Can you work these out from the model? Positions are in its coordinate system, mm. A direction names the side the tool comes from. Round coordinates to 2 decimals unless told otherwise and drop trailing zeros. Write each loop counter-clockwise with the first axis right and the second up, starting at its lowest first coordinate (ties: lowest second). Pieces come first, ordered by that corner, then holes.
Q1. Please list where these lines run through material, in increasing order: line 1 along Z through (x, y) = (-3.5, -0.5); line 2 along Z through (x, y) = (-2, -2); line 3 along Y through (x, z) = (8.5, -5) (3 decimals).
Q2. For faces 1 (the cylindrical face through (-7.81, 13.27, -1.73)), 2 (the flat face through (26.924, 0, 0)), 3 (the cylindrical face through (13.27, -7.81, 1.73)), which set-ups out of +Z, -Z, +X, -X, +Y, -Y let a thin tool reach every point of the face, with its end or its side?
Q3. If we section it at A-A (z = 0): Please give me the cut outline in (x, y).
Q4. If we section it at D-D (z = -3): Please give me the cut outline in (x, y).
Q5. If we section it at B-B (x = 21): Please give me the cut outline in (y, z).
Q6. I'm going to push flat-ended pins straight in: pin 1 Ø2 at (x, z) = (7, -4.5) entering from -Y; pin 2 Ø1 at (x, z) = (20.5, -2) entering from +Y; pin 3 Ø1.5 at (x, z) = (7, -6) entering from -Y. Where does each tip first touch, or does it pass through?
from build123d import *

# Parameters (mm, degrees)
SKETCH1_R           = 8
BOSS_EXTRUDE1_DEPTH = 26.924
SKETCH2_R           = 8
BOSS_EXTRUDE2_DEPTH = 26.924
REVOLVE1_ANGLE      = 90


with BuildPart() as part:
    # Sketch1 → Boss-Extrude1 (new body)
    with BuildSketch(Plane(origin=(0, 0, 0), x_dir=(1, 0, 0), z_dir=(0, 1, 0))):
        with Locations(Location((0, 0, 0), (0, 0, 270))):
            Circle(SKETCH1_R)
    extrude(amount=BOSS_EXTRUDE1_DEPTH)

    # Sketch2 → Boss-Extrude2 (add)
    with BuildSketch(Plane(origin=(0, 0, 0), x_dir=(0, 0, -1), z_dir=(1, 0, 0))):
        Circle(SKETCH2_R)
    extrude(amount=BOSS_EXTRUDE2_DEPTH)

    # Sketch3 → Revolve1 (revolve)
    with BuildSketch(Plane.ZY):
        with BuildLine():
            Line((-8, 0), (8, 0))
            ThreePointArc((8, 0), (0, -8), (-8, 0))
        make_face()
    revolve(axis=Axis((0, 0, 0), (0, 0, -1)), revolution_arc=REVOLVE1_ANGLE)


solid = part.part
A:
1. line 1: z = -7.18 to 7.18
1. line 2: z = -7.48 to 7.48
1. line 3: y = -6.245 to 6.245
2. face 1: +Y
2. face 2: +Z, -Z, +X, +Y, -Y
2. face 3: +X
3. outline: (-8, 0) arc R8 ccw to (0, -8) - (26.92, -8) - (26.92, 8) - (8, 8) - (8, 26.92) - (-8, 26.92) - close
4. outline: (-7.42, 0) arc R7.42 ccw to (0, -7.42) - (26.92, -7.42) - (26.92, 7.42) - (7.42, 7.42) - (7.42, 26.92) - (-7.42, 26.92) - close
5. outline: circle Ø16 at (0, 0)
6. pin 1: stops at y = -7.19
6. pin 2: stops at y = 7.86
6. pin 3: stops at y = -6.04
